Part model, mm, in its own coordinate system. A direction names the side the tool comes from. Round coordinates to 2 decimals unless told otherwise and drop trailing zeros. Write each loop counter-clockwise with the first axis right and the second up, starting at its lowest first coordinate (ties: lowest second). Pieces come first, ordered by that corner, then holes. Notation, with made-up numbers: M 81,21 L 116,21 A22 cw 116,38 Z; hole C 65,13.25 d2. An arc over 180 degrees is marked long. Answer as a JSON object with one key per item and string values. Group by question number.
1. Band-saw the part on A-A, the plane x = 0.5. Write the cut outline in (y, z).
2. Which spindle directions (+Z, -Z, +X, -X, +Y, -Y) get a long thin tool onto all of the face, cutting with end or side? Do faces 4 (the face through (0, -20, 6)), 5 (the face through (0, -20, 4)), 6 (the face through (20, 10, 6)), 7 (the face through (-14, -13.262, 5)). Say none if no direction does.
3. Two-plate mould, pull along Y, no slides. Class faces 1 (the face through (18, 4.238, 5)), 2 (the face through (-5.436, -21, 5)), 3 (the face through (-14, -10, 6.25)): +Y half, -Y half, draft (parallel to the pull), parting line (faces both ways), or undercut.
4. Band-saw the part on C-C, the plane x = 13.5. Write the cut outline in (y, z).
5. Drop flat-ended pins along their axis: pin 1 (1.1 mm diameter, centred on x = -14.5, z = 5.5, fed in from -Y); pin 2 (1.5 mm diameter, centred on x = 7.5, z = 5, fed in from +Y); pin 3 (3 mm diameter, centred on x = -1.5, y = -21, fed in from -Z). Give the stop position or say it passes through.
6. Drill centre lines: line 1 (X direction, y = 17.4, z = 5); line 2 (Y direction, x = -14, z = 5.5); line 3 (Y direction, x = -13.5, z = 1). Where is each one in solid material? Low to high. Write a range as from..to.
7. Band-saw the part on B-B, the plane y = -12.5. Write the cut outline in (x, z).
8. Band-saw the part on D-D, the plane y = -5. Write the cut outline in (x, z).
from build123d import *

# Parameters (mm, degrees)
SKETCH1_W           = 30
SKETCH1_H           = 34.5
BOSS_EXTRUDE1_DEPTH = 10
SKETCH2_W           = 2
SKETCH2_H           = 11.5
BOSS_EXTRUDE4_DEPTH = 21
SKETCH3_W           = 11.5
SKETCH3_H           = 2
BOSS_EXTRUDE5_DEPTH = 6
FILLET2_R           = 1
SKETCH4_R           = 1.375
CUT_EXTRUDE1_DEPTH  = 10
FILLET3_R           = 0.5
SKETCH5_W           = 2.5
SKETCH5_H           = 6
CUT_EXTRUDE2_DEPTH  = 1
SKETCH6_R           = 3
SKETCH6_R_2         = 1
BOSS_EXTRUDE6_DEPTH = 3
CUT_EXTRUDE3_START  = -3
CUT_EXTRUDE3_DEPTH  = 3
CIRPATTERN1_COUNT   = 24


with BuildPart() as part:
    # Sketch1 → Boss-Extrude1 (new body)
    with BuildSketch(Plane.XY):
        with Locations((0.31359995, -1.512440758)):
            Rectangle(SKETCH1_W, SKETCH1_H)
    extrude(amount=BOSS_EXTRUDE1_DEPTH)

    # Sketch2 → Boss-Extrude4 (add, symmetric)
    with BuildSketch(Plane(origin=(0.31359995, 0, 0), x_dir=(0, 0, -1), z_dir=(1, 0, 0))):
        with Locations((-5, 9.987559242)):
            Rectangle(SKETCH2_W, SKETCH2_H)
    extrude(amount=BOSS_EXTRUDE4_DEPTH, both=True)

    # Sketch3 → Boss-Extrude5 (add)
    with BuildSketch(Plane.XZ.offset(18.762440758)):
        with Locations((0.31359995, 5)):
            Rectangle(SKETCH3_W, SKETCH3_H)
    extrude(amount=BOSS_EXTRUDE5_DEPTH)

    # Fillet2
    fillet2_edges = [part.edges().sort_by_distance(p)[0] for p in [
        (21.31359995, 15.737559242, 5),
        (-20.68640005, 4.237559242, 5),
        (21.31359995, 4.237559242, 5),
        (-20.68640005, 15.737559242, 5),
        (-5.43640005, -24.762440758, 5),
        (6.06359995, -24.762440758, 5),
    ]]
    fillet(fillet2_edges, radius=FILLET2_R)

    # Sketch4 → Cut-Extrude1 (cut)
    with BuildSketch(Plane.XY.offset(10)):
        with Locations((-17.68640005, 9.987559242)):
            Circle(SKETCH4_R)
        with Locations((18.31359995, 9.987559242)):
            Circle(SKETCH4_R)
        with Locations((0.31359995, -21.762440758)):
            Circle(SKETCH4_R)
    extrude(amount=-CUT_EXTRUDE1_DEPTH, mode=Mode.SUBTRACT)

    # Fillet3
    fillet3_edges = [part.edges().sort_by_distance(p)[0] for p in [
        (15.31359995, -1.512440758, 10),
        (-14.68640005, -1.512440758, 10),
        (15.31359995, -1.512440758, 0),
        (0.31359995, -18.762440758, 0),
        (-14.68640005, -1.512440758, 0),
        (15.31359995, -18.762440758, 5),
        (-14.68640005, -18.762440758, 5),
        (0.31359995, -18.762440758, 10),
    ]]
    fillet(fillet3_edges, radius=FILLET3_R)

    # Sketch5 → Cut-Extrude2 (cut)
    with BuildSketch(Plane.ZY.offset(14.68640005)):
        with Locations((5, -10.262440758)):
            Rectangle(SKETCH5_W, SKETCH5_H)
    extrude(amount=-CUT_EXTRUDE2_DEPTH, mode=Mode.SUBTRACT)

    # Sketch6 → Boss-Extrude6 (add)
    with BuildSketch(Plane(origin=(0, 15.737559242, 0), x_dir=(1, 0, 0), z_dir=(0, 1, 0))):
        with Locations(Location((-9.68640005, -5, 0), (0, 0, 90))):
            Circle(SKETCH6_R)
        with Locations(Location((-9.68640005, -5, 0), (0, 0, 270))):
            Circle(SKETCH6_R_2, mode=Mode.SUBTRACT)
    extrude(amount=BOSS_EXTRUDE6_DEPTH)

    # Sketch7 → Cut-Extrude3 (cut)
    with BuildSketch(Plane(origin=(0, 18.737559242, 0), x_dir=(1, 0, 0), z_dir=(0, 1, 0)).offset(CUT_EXTRUDE3_START)):
        with BuildLine():
            Line((-9.68640005, -2), (-9.68640005, -2.5))
            Line((-9.68640005, -2.5), (-9.61140005, -2.5))
            ThreePointArc((-9.61140005, -2.5), (-9.571129509, -2.240512735), (-9.446003633, -2.009647251))
            ThreePointArc((-9.446003633, -2.009647251), (-9.566105093, -2.002412783), (-9.68640005, -2))
        make_face()
        with BuildLine():
            Line((-9.76140005, -2.5), (-9.68640005, -2.5))
            Line((-9.68640005, -2.5), (-9.68640005, -2))
            ThreePointArc((-9.68640005, -2), (-9.806695006, -2.002412783), (-9.926796466, -2.009647251))
            ThreePointArc((-9.926796466, -2.009647251), (-9.80167059, -2.240512735), (-9.76140005, -2.5))
        make_face()
    cut_extrude3 = extrude(amount=CUT_EXTRUDE3_DEPTH, mode=Mode.SUBTRACT)

    # CirPattern1: Cut-Extrude3 ×24 about axis
    cirpattern1_axis = Axis((-9.68640005, 0, 5), (0, 1, 0))
    for i in range(1, CIRPATTERN1_COUNT):
        add(cut_extrude3.rotate(cirpattern1_axis, i * 360 / CIRPATTERN1_COUNT), mode=Mode.SUBTRACT)


solid = part.part
Worked answers:
{
 "1": {"outline": "M -24.76,4 L -23.12,4 L -23.12,6 L -24.76,6 Z; M -20.4,4 L -18.76,4 L -18.76,0.5 A0.5 ccw -18.26,0 L 15.74,0 L 15.74,10 L -18.26,10 A0.5 ccw -18.76,9.5 L -18.76,6 L -20.4,6 Z"},
 "2": {"face 4": "+Z, +X, -X, -Y", "face 5": "-Z, +X, -X, -Y", "face 6": "+Z, +X, +Y, -Y", "face 7": "-X"},
 "3": {"face 1": "-Y half", "face 2": "draft", "face 3": "undercut"},
 "4": {"outline": "M -18.76,0.5 A0.5 ccw -18.26,0 L 15.74,0 L 15.74,10 L -18.26,10 A0.5 ccw -18.76,9.5 Z"},
 "5": {"pin 1": "stops at y = -18.76", "pin 2": "stops at y = 15.74", "pin 3": "stops at z = 4"},
 "6": {"line 1": "x = -12.19..-10.69, -8.69..-7.19", "line 2": "y = -18.76..-13.26, -7.26..15.74", "line 3": "y = -18.76..15.74"},
 "7": {"outline": "M -14.69,0.5 A0.5 ccw -14.19,0 L 14.81,0 A0.5 ccw 15.31,0.5 L 15.31,9.5 A0.5 ccw 14.81,10 L -14.19,10 A0.5 ccw -14.69,9.5 L -14.69,6.25 L -13.69,6.25 L -13.69,3.75 L -14.69,3.75 Z"},
 "8": {"outline": "M -14.69,0.5 A0.5 ccw -14.19,0 L 14.81,0 A0.5 ccw 15.31,0.5 L 15.31,9.5 A0.5 ccw 14.81,10 L -14.19,10 A0.5 ccw -14.69,9.5 Z"}
}
